from build123d import *

# Parameters (mm, degrees)
ESQUISSE1_W             = 75
ESQUISSE1_H             = 63
BOSS_EXTRU_1_DEPTH      = 800
ESQUISSE2_R             = 5
ENL_V_MAT_EXTRU_1_DEPTH = 806.973944988
ESQUISSE3_W             = 75
ESQUISSE3_H             = 63
ENL_V_MAT_EXTRU_2_DEPTH = 20


with BuildPart() as part:
    # Esquisse1 → Boss.-Extru.1 (new body)
    with BuildSketch(Plane.XY):
        with Locations((37.5, 31.5)):
            Rectangle(ESQUISSE1_W, ESQUISSE1_H)
    extrude(amount=BOSS_EXTRU_1_DEPTH)

    # Esquisse2 → Enlèv. mat.-Extru.1 (cut, through all)
    with BuildSketch(Plane.XZ):
        with Locations(Location((19, 752, 0), (0, 0, 270))):
            Circle(ESQUISSE2_R)
        with Locations(Location((19, 785, 0), (0, 0, 270))):
            Circle(ESQUISSE2_R)
        with Locations(Location((56, 785, 0), (0, 0, 90))):
            Circle(ESQUISSE2_R)
        with Locations(Location((56, 752, 0), (0, 0, 90))):
            Circle(ESQUISSE2_R)
    extrude(amount=-ENL_V_MAT_EXTRU_1_DEPTH, mode=Mode.SUBTRACT)

    # Esquisse3 → Enlèv. mat.-Extru.2 (cut)
    with BuildSketch(Plane.XZ):
        with Locations((37.5, 181.5)):
            Rectangle(ESQUISSE3_W, ESQUISSE3_H)
    extrude(amount=-ENL_V_MAT_EXTRU_2_DEPTH, mode=Mode.SUBTRACT)


solid = part.part
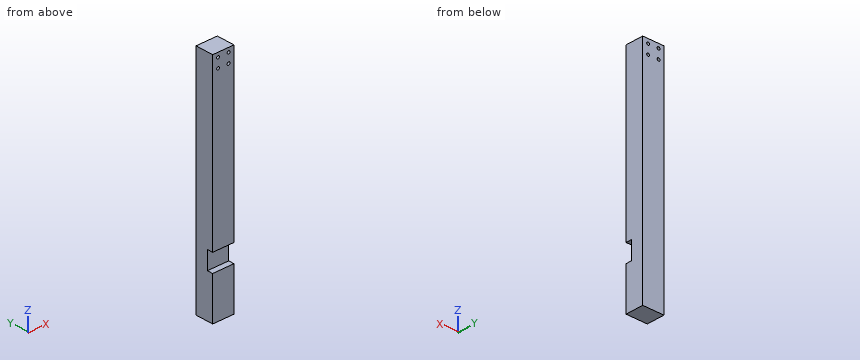
Part model, mm, in its own coordinate system. Round coordinates to 2 decimals unless told otherwise and drop trailing zeros. Loops run counter-clockwise (first coordinate to the right, second up) from the corner with the lowest first, then second, coordinate; pieces in that order, holes last. Notation, with made-up numbers: (-7.75, 25.25) - (16.25, 25.25) arc R13 ccw to (16.25, 50.25) - close; hole circle Ø10 at (-35.5, 84). An arc over 180 degrees is marked (long way). Answer as a JSON object with one key per item and string values.
Item 1: Band-saw the part on A-A on y = 13.5. List the corners of the cut face in (x, z).
Output:
{"outline": "(0, 0) - (75, 0) - (75, 150) - (0, 150) - close; (0, 213) - (75, 213) - (75, 800) - (0, 800) - close; hole circle Ø10 at (19, 752); hole circle Ø10 at (19, 785); hole circle Ø10 at (56, 752); hole circle Ø10 at (56, 785)"}
Item 2: Band-saw the part on B-B on x = 43. List the corners of the cut face in (y, z).
Output:
{"outline": "(0, 0) - (63, 0) - (63, 800) - (0, 800) - (0, 213) - (20, 213) - (20, 150) - (0, 150) - close"}
Item 3: Wall check: L1, parallel to X at y = 37, z = 785; L2, parallel to Z at x = 56, y = 30; L3, parallel to Z at x = 70, y = 15.5. Give the ranges that are in metal, low to high.
Output:
{"L1": "0 to 14, 24 to 51, 61 to 75", "L2": "0 to 747, 757 to 780, 790 to 800", "L3": "0 to 150, 213 to 800"}
Item 4: Pin check, flat tip, straight feed: pin 1 (6 mm diameter, centred on x = 19, z = 752, fed in from -Y). Stop position of the tip, or through.
Output:
{"pin 1": "through"}
Item 5: Band-saw the part on C-C on z = 194.5. List the corners of the cut face in (x, y), plus the area to 4 significant figures.
Output:
{"outline": "(0, 20) - (75, 20) - (75, 63) - (0, 63) - close", "area": "3,225 mm2"}
